```python
from build123d import *

# Parameters (mm, degrees)
PAD_DEPTH    = 3.4
SKETCH001_R  = 1.6
POCKET_DEPTH = 3.5


with BuildPart() as part:
    # Sketch → Pad (new body, symmetric)
    with BuildSketch(Plane.XY):
        with BuildLine():
            ThreePointArc((3.5, -4.5), (4.56066, -4.06066), (5, -3))
            Line((5, 3), (5, -3))
            ThreePointArc((5, 3), (4.56066, 4.06066), (3.5, 4.5))
            Line((3.5, 4.5), (0, 4.5))
            Line((0, 4.5), (0, -4.5))
            Line((0, -4.5), (3.5, -4.5))
        make_face()
    extrude(amount=PAD_DEPTH, both=True)

    # Sketch001 (on Face5 of Pad) → Pocket (cut)
    with BuildSketch(Plane(origin=(0, 0, 0), x_dir=(0, -1, 0), z_dir=(-1, 0, 0))):
        Circle(SKETCH001_R)
    extrude(amount=-POCKET_DEPTH, mode=Mode.SUBTRACT)


solid = part.part
```
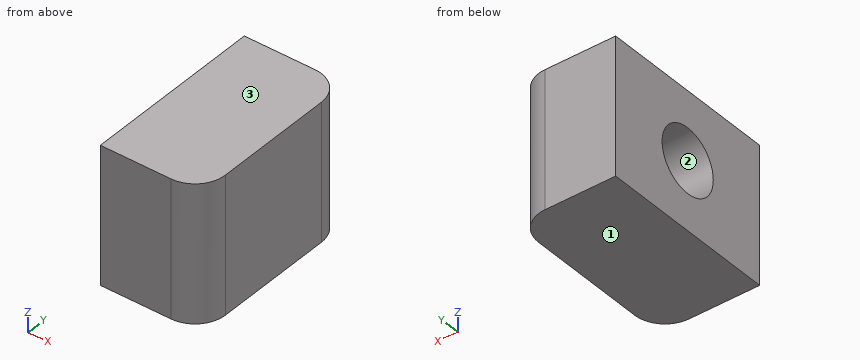
Geometry: final body of the model. Coordinates: model frame, mm. Face numbers are marked on the shaded views. Round coordinates to 2 decimals unless told otherwise and drop trailing zeros. Write each loop counter-clockwise with the first axis right and the second up, starting at its lowest first coordinate (ties: lowest second). Pieces come first, ordered by that corner, then holes.
Item 1: Section query A-A (y = 0). Return loops of the section in (x, z).
Item 2: Section query C-C (z = 0). Return loops of the section in (x, y), plus the area to 3 significant figures.
Item 3: Section query D-D (x = 4.4). Return loops of the section in (y, z), plus the area to 3 significant figures.
Item 4: Mould query, pull axis Z, two halves, no side actions, for the marked faces 1, 2 and 3. Classes: +Z half, -Z half, draft (parallel to the pull), parting line (faces both ways), or undercut.
Item 5: Material intervals for L1, parallel to Z at x = 1.4, y = 0; L2, parallel to X at y = 0, z = 1.5; L3, parallel to Y at x = 2.45, z = -0.5, sorted ascending.
Item 6: Section query B-B (x = 2.8). Return loops of the section in (y, z).
Completed:
1. outline: (0, -3.4) - (5, -3.4) - (5, 3.4) - (0, 3.4) - (0, 1.6) - (3.5, 1.6) - (3.5, -1.6) - (0, -1.6) - close
2. outline: (0, -4.5) - (3.5, -4.5) arc R1.5 ccw to (5, -3) - (5, 3) arc R1.5 ccw to (3.5, 4.5) - (0, 4.5) - (0, 1.6) - (3.5, 1.6) - (3.5, -1.6) - (0, -1.6) - close
2. area: 32.8 mm2
3. outline: (-4.2, -3.4) - (4.2, -3.4) - (4.2, 3.4) - (-4.2, 3.4) - close
3. area: 57.1 mm2
4. face 1: -Z half
4. face 2: undercut
4. face 3: +Z half
5. L1: z = -3.4 to -1.6, 1.6 to 3.4
5. L2: x = 3.5 to 5
5. L3: y = -4.5 to -1.52, 1.52 to 4.5
6. outline: (-4.5, -3.4) - (4.5, -3.4) - (4.5, 3.4) - (-4.5, 3.4) - close; hole circle Ø3.2 at (0, 0)
